Geometry: final body of the model. Coordinates: model frame, mm. Face numbers are marked on the shaded views. A direction names the side the tool comes from. Give positions to 0.01 mm unless a question says otherwise; leave off trailing zeros. Order: outer loops, then holes, each group sorted by start corner. A loop starts at its lowest first (then second) coordinate and runs counter-clockwise, first axis right, second up. Notation, with made-up numbers: (39.25, 25) -> (90.25, 25) arc R16 cw to (90.25, 31) -> close; hole circle Ø4 at (11.25, 60.5). An arc over 180 degrees is marked (long way). Write item = value, one per line.
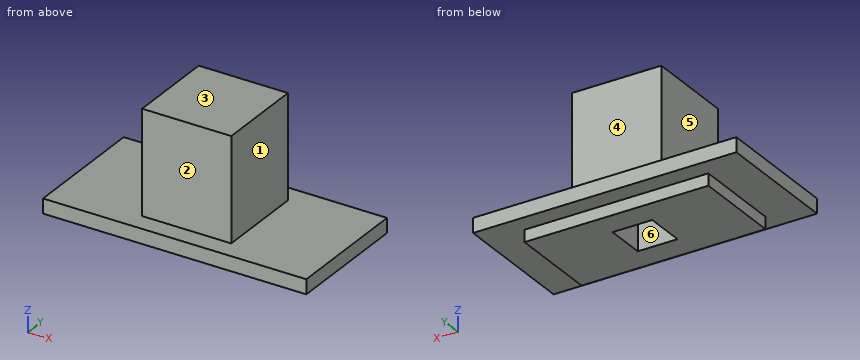
```python
from build123d import *

# Parameters (mm, degrees)
F0_W     = 9.95
F0_H     = 4.8
F1_DEPTH = 0.55
F2_W     = 6.95
F2_H     = 3.4
F3_DEPTH = 0.45
F4_W     = 3.37
F4_H     = 3.37
F5_DEPTH = 3.91
F6_W     = 1.5
F6_H     = 1.5
F7_DEPTH = 4.5


with BuildPart() as f1:
    # F0 (on Top) → F1 (new body)
    with BuildSketch(Plane.XY):
        with Locations((4.975, 2.4)):
            Rectangle(F0_W, F0_H)
    extrude(amount=-F1_DEPTH)

    # F2 (on face) → F3 (join)
    with BuildSketch(Plane(origin=(0, 0, -0.55), x_dir=(1, 0, 0), z_dir=(0, 0, -1))):
        with Locations((4.975, -2.4)):
            Rectangle(F2_W, F2_H)
    extrude(amount=F3_DEPTH)

    # F4 (on face) → F5 (join)
    with BuildSketch(Plane.XY):
        with Locations((4.975, 2.4)):
            Rectangle(F4_W, F4_H)
    extrude(amount=F5_DEPTH)

    # F6 (on face) → F7 (cut)
    with BuildSketch(Plane(origin=(0, 0, -1), x_dir=(1, 0, 0), z_dir=(0, 0, -1))):
        with Locations((4.975, -2.4)):
            Rectangle(F6_W, F6_H)
    extrude(amount=-F7_DEPTH, mode=Mode.SUBTRACT)


solid = f1.part
```
1) Section query A-A (z = -0.65). Output: boundary loops of the cut face in (x, y) (3 decimals), plus the area to 3 significant figures.
Check sheet entries:
outline = (1.5, 0.7) -> (8.45, 0.7) -> (8.45, 4.1) -> (1.5, 4.1) -> close; hole (4.225, 1.65) -> (5.725, 1.65) -> (5.725, 3.15) -> (4.225, 3.15) -> close
area = 21.4 mm²
2) Mould query, pull axis X, two halves, no side actions, for the marked faces 4, 5 and 6. Classes: +X half, -X half, draft (parallel to the pull), parting line (faces both ways), or undercut.
Check sheet entries:
face_4 = draft
face_5 = -X half
face_6 = undercut
3) Section query D-D (z = 0.25). Output: boundary loops of the cut face in (x, y) (3 decimals).
Check sheet entries:
outline = (3.29, 0.715) -> (6.66, 0.715) -> (6.66, 4.085) -> (3.29, 4.085) -> close; hole (4.225, 1.65) -> (5.725, 1.65) -> (5.725, 3.15) -> (4.225, 3.15) -> close
4) First-contact query: P1, Ø0.8, axis at x = 5, z = 2.5, coming from the -Y side (3 decimals); P2, Ø0.8, axis at x = 5, z = 2.5, coming from the +Y side (3 decimals); P3, Ø2.5, axis at y = 3, z = 2, coming from the -X side. Flat tips, straight axial feed; report the tip coordinate or a pass-through.
Check sheet entries:
P1 = 0.715
P2 = 4.085
P3 = 3.29
5) Reachability of the marked faces 1, 2 and 3 from +Z, -Z, +X, -X, +Y, -Y: full face, straight path, thin tool, end or side. Return the list, or none.
Check sheet entries:
face_1 = +Z, +X, +Y, -Y
face_2 = +Z, +X, -X, -Y
face_3 = +Z, +X, -X, +Y, -Y
6) Section query C-C (x = 3.5). Output: boundary loops of the cut face in (y, z) (3 decimals), plus the area to 3 significant figures.
Check sheet entries:
outline = (0, -0.55) -> (0.7, -0.55) -> (0.7, -1) -> (4.1, -1) -> (4.1, -0.55) -> (4.8, -0.55) -> (4.8, 0) -> (4.085, 0) -> (4.085, 3.91) -> (0.715, 3.91) -> (0.715, 0) -> (0, 0) -> close
area = 17.3 mm²
7) Line query: line 1 (Y direction, x = 4.75, z = 0.7) (3 decimals); line 2 (X direction, y = 3.1, z = 0.25) (3 decimals); line 3 (X direction, y = 3.9, z = 2.9). Output: solid intervals per line, ascending. Write a range as from..to.
Check sheet entries:
line_1 = 0.715..1.65, 3.15..4.085
line_2 = 3.29..4.225, 5.725..6.66
line_3 = 3.29..6.66
8) Section query B-B (y = 2.3). Output: boundary loops of the cut face in (x, z) (3 decimals).
Check sheet entries:
outline = (0, -0.55) -> (1.5, -0.55) -> (1.5, -1) -> (4.225, -1) -> (4.225, 3.5) -> (5.725, 3.5) -> (5.725, -1) -> (8.45, -1) -> (8.45, -0.55) -> (9.95, -0.55) -> (9.95, 0) -> (6.66, 0) -> (6.66, 3.91) -> (3.29, 3.91) -> (3.29, 0) -> (0, 0) -> close
